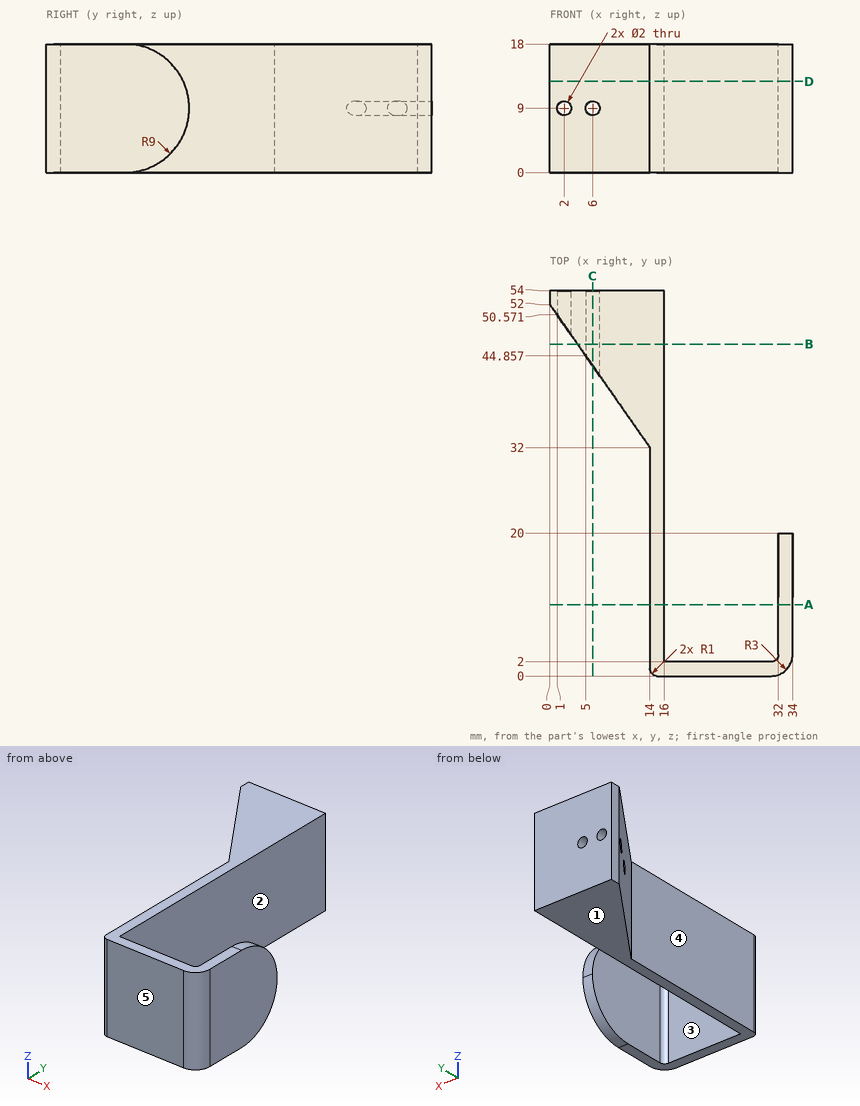
The drawing under review shows one solid part. Ordinate dimensions are in mm from its lowest x, y, z. A direction names the side the tool comes from. Coordinates: 2 decimals unless noted, no trailing zeros. Loops run counter-clockwise (first coordinate to the right, second up) from the corner with the lowest first, then second, coordinate; pieces in that order, holes last. Notation, with made-up numbers: (6.5, 35) -> (20.5, 35) arc R16 ccw to (20.5, 44) -> close; hole circle Ø5 at (85.5, 63). An arc over 180 degrees is marked (long way). Answer as a JSON object with one key per item and string values.
Q1. Tool access review of the marked faces 1 and 2: name each direction out of +Z, -Z, +X, -X, +Y, -Y from which nothing blocks a thin tool from reaching the whole face with its end or side.
Answer block:
{"face 1": "-Z, +X, -X, +Y, -Y", "face 2": "+Z, -Z, +Y"}
Q2. Clearance check with flat-ended pins moving along their axes: pin 1 Ø1.8 at (x, z) = (2, 9) entering from -Y; pin 2 Ø2 at (y, z) = (12, 7.5) entering from -X; pin 3 Ø4.5 at (x, z) = (25.5, 8.5) entering from +Y; pin 4 Ø3 at (x, z) = (4, 15.5) entering from -Y (1 decimal). State where each tip first meets the part, or that it passes through.
Answer block:
{"pin 1": "passes through", "pin 2": "stops at x = 14", "pin 3": "stops at y = 2", "pin 4": "stops at y = 44.1"}
Q3. Take a section at B-B on y = 46.5. Give the boundary of the cut face in (x, z), plus the area to 3 significant figures.
Answer block:
{"outline": "(3.85, 0) -> (16, 0) -> (16, 18) -> (3.85, 18) -> close; hole circle Ø2 at (6, 9)", "area": "216 mm^2"}
Q4. Take a section at C-C on x = 6. Give the boundary of the cut face in (y, z), plus the area to 3 significant figures.
Answer block:
{"outline": "(43.43, 0) -> (54, 0) -> (54, 8) -> (43.43, 8) -> close; (43.43, 10) -> (54, 10) -> (54, 18) -> (43.43, 18) -> close", "area": "169 mm^2"}
Q5. Take a section at A-A on y = 10. Give the boundary of the cut face in (x, z).
Answer block:
{"outline": "(14, 0) -> (16, 0) -> (16, 18) -> (14, 18) -> close; (32, 0) -> (34, 0) -> (34, 18) -> (32, 18) -> close"}
Q6. To check wall thickness, follow L1, parallel to Z at x = 2, y = 50; L2, parallel to X at y = 11.5, z = 5.75; L3, parallel to Y at x = 27, z = 14.5. State the ranges of each line that lie inside material, in increasing order.
Answer block:
{"L1": "z = 0 to 8, 10 to 18", "L2": "x = 14 to 16, 32 to 34", "L3": "y = 0 to 2"}
Q7. The part is to be moulded in two halves that separate along X. For the marked faces 3, 4 and 5, say which applies: +X half, -X half, draft (parallel to the pull), parting line (faces both ways), or undercut.
Answer block:
{"face 3": "undercut", "face 4": "-X half", "face 5": "draft"}
Q8. Take a section at D-D on z = 12.75. Give the boundary of the cut face in (x, y).
Answer block:
{"outline": "(0, 52) -> (14, 32) -> (14, 1) arc R1 ccw to (15, 0) -> (31, 0) arc R3 ccw to (34, 3) -> (34, 19.18) -> (32, 19.18) -> (32, 3) arc R1 cw to (31, 2) -> (16, 2) -> (16, 54) -> (0, 54) -> close"}
